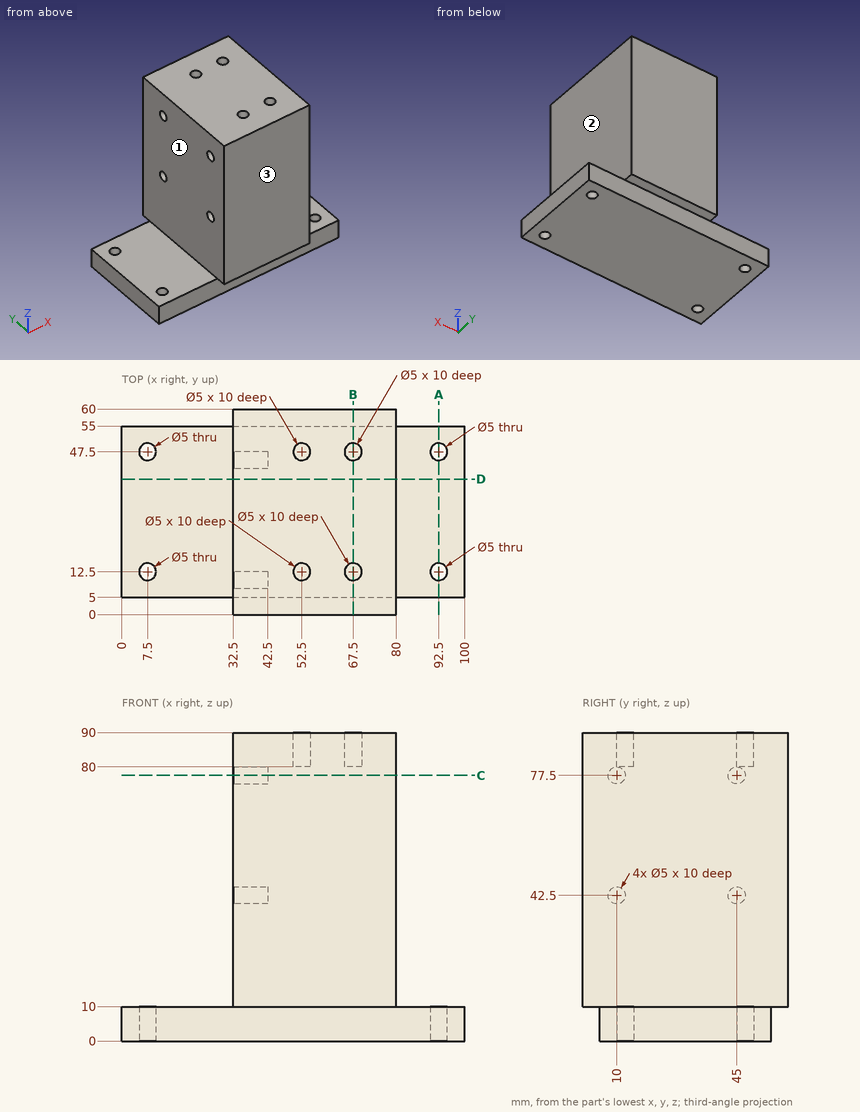
Part print with two shaded views. Sizes in mm from the minimum x, y, z corner. A direction names the side the tool comes from. Give positions to 0.01 mm unless a question says otherwise; leave off trailing zeros. Order: outer loops, then holes, each group sorted by start corner. A loop starts at its lowest first (then second) coordinate and runs counter-clockwise, first axis right, second up.
1) Pin check, flat tips, straight feed: pin 1 (5 mm diameter, centred on y = 49.5, z = 43, fed in from +X); pin 2 (4 mm diameter, centred on y = 44.5, z = 42, fed in from -X); pin 3 (8 mm diameter, centred on x = 69, z = 3.5, fed in from -Y). Stop position of each tip, or through.
2) Saw through at C-C, the plane z = 77.5. Write the cut outline in (x, y).
3) Saw through at A-A, the plane x = 92.5. Write the cut outline in (y, z), then the cut area to 3 significant figures.
4) 3-axis set-ups, long thin cutter, end or side, ignore diameter. For the marked faces 1, 2 and 3: which of +Z, -Z, +X, -X, +Y, -Y reach the whole face in a straight line?
5) Wall check: probe 1 along Y at (x, z) = (39, 42.5); probe 2 along Y at (x, z) = (52.5, 85.5); probe 3 along X at (y, z) = (12, 5). Give the ranges that are in metal, low to high.
6) Saw through at B-B, the plane x = 67.5. Write the cut outline in (y, z), then the cut area to 3 significant figures.
7) Saw through at D-D, the plane y = 39.5. Write the cut outline in (x, z), then the cut area to 3 significant figures.
Computed:
1. pin 1: stops at x = 80
1. pin 2: stops at x = 32.5
1. pin 3: stops at y = 5
2. outline: (32.5, 0) - (80, 0) - (80, 60) - (32.5, 60) - (32.5, 47.5) - (42.5, 47.5) - (42.5, 42.5) - (32.5, 42.5) - (32.5, 12.5) - (42.5, 12.5) - (42.5, 7.5) - (32.5, 7.5) - close
3. outline: (5, 0) - (10, 0) - (10, 10) - (5, 10) - close; (15, 0) - (45, 0) - (45, 10) - (15, 10) - close; (50, 0) - (55, 0) - (55, 10) - (50, 10) - close
3. area: 400 mm2
4. face 1: +Z, -X, +Y, -Y
4. face 2: +Z, +X, +Y, -Y
4. face 3: +Z, -Z, +X, -X, -Y
5. probe 1: y = 0 to 7.5, 12.5 to 42.5, 47.5 to 60
5. probe 2: y = 0 to 10, 15 to 45, 50 to 60
5. probe 3: x = 0 to 5.05, 9.95 to 90.05, 94.95 to 100
6. outline: (0, 10) - (5, 10) - (5, 0) - (55, 0) - (55, 10) - (60, 10) - (60, 90) - (50, 90) - (50, 80) - (45, 80) - (45, 90) - (15, 90) - (15, 80) - (10, 80) - (10, 90) - (0, 90) - close
6. area: 5,200 mm2
7. outline: (0, 0) - (100, 0) - (100, 10) - (80, 10) - (80, 90) - (32.5, 90) - (32.5, 10) - (0, 10) - close
7. area: 4,800 mm2
